from build123d import *

# Parameters (mm, degrees)
SKETCH1_R                = 2.15
BOSS_EXTRUDE1_DEPTH      = 8
BOSS_EXTRUDE2_START      = -4
BOSS_EXTRUDE2_DEPTH      = 4
SKETCH3_W                = 56
SKETCH3_H                = 8
BOSS_EXTRUDE6_DEPTH      = 7
BOSS_EXTRUDE4_START      = -8
BOSS_EXTRUDE4_DEPTH      = 8
CUT_EXTRUDE1_DEPTH       = 67.44206881
FILLET4_R                = 8
FILLET3_R                = 4
M3_CLEARANCE_HOLE1_D     = 3.2
M3_CLEARANCE_HOLE1_DEPTH = 8
M3_CLEARANCE_HOLE1_TIP   = 0.96137699


with BuildPart() as part:
    # Sketch1 → Boss-Extrude1 (new body)
    with BuildSketch(Plane.XY):
        with BuildLine():
            Line((-46, 10), (46, 10))
            ThreePointArc((46, 10), (56, 0), (46, -10))
            Line((46, -10), (-46, -10))
            ThreePointArc((-46, -10), (-56, 0), (-46, 10))
        make_face()
        with Locations((-46, 0)):
            Circle(SKETCH1_R, mode=Mode.SUBTRACT)
        with Locations((46, 0)):
            Circle(SKETCH1_R, mode=Mode.SUBTRACT)
    extrude(amount=BOSS_EXTRUDE1_DEPTH)

    # Sketch2 → Boss-Extrude2 (add)
    with BuildSketch(Plane.XY.offset(8).offset(BOSS_EXTRUDE2_START)):
        with BuildLine():
            Line((-46, -10), (46, -10))
            ThreePointArc((46, -10), (56, 0), (46, 10))
            Line((46, 10), (-46, 10))
            ThreePointArc((-46, 10), (-56, 0), (-46, -10))
        make_face()
    extrude(amount=BOSS_EXTRUDE2_DEPTH)

    # Sketch3 → Boss-Extrude6 (add)
    with BuildSketch(Plane(origin=(0, 10, 0), x_dir=(1, 0, 0), z_dir=(0, 1, 0))):
        with Locations((0, -4)):
            Rectangle(SKETCH3_W, SKETCH3_H)
    extrude(amount=BOSS_EXTRUDE6_DEPTH)

    # Sketch4 → Boss-Extrude4 (add)
    with BuildSketch(Plane.XY.offset(8).offset(BOSS_EXTRUDE4_START)):
        with BuildLine():
            Line((-46, -10), (46, -10))
            ThreePointArc((46, -10), (50.753025174, -8.798224349), (54.363636364, -5.481750339))
            ThreePointArc((54.363636364, -5.481750339), (0, -34.850373137), (-54.363636364, -5.481750339))
            ThreePointArc((-54.363636364, -5.481750339), (-50.753025174, -8.798224349), (-46, -10))
        make_face()
    extrude(amount=BOSS_EXTRUDE4_DEPTH)

    # Sketch5 → Cut-Extrude1 (cut, through all)
    with BuildSketch(Plane(origin=(0, 0, 0), x_dir=(-1, 0, 0), z_dir=(0, 0, -1))):
        with BuildLine():
            Line((-20.322585041, 0), (20.322585041, 0))
            ThreePointArc((20.322585041, 0), (30.049388036, -7.678512657), (24.83871505, -18.922139303))
            ThreePointArc((24.83871505, -18.922139303), (0, -24.850373137), (-24.83871505, -18.922139303))
            ThreePointArc((-24.83871505, -18.922139303), (-30.049388036, -7.678512657), (-20.322585041, 0))
        make_face()
    extrude(amount=-CUT_EXTRUDE1_DEPTH, mode=Mode.SUBTRACT)

    # Fillet4
    # the kernel refuses this fillet: 8 mm, written as the material it adds along each edge
    with BuildSketch(Plane(origin=(28, 10, 8), x_dir=(0, 1, 0), z_dir=(0, 0, -1))) as fillet4_piece_1:
        with BuildLine():
            CenterArc((8, 7.937253933), FILLET4_R, 180, 82.819244219)
            Line((0, 7.937253933), (-0.16, 7.937253933))
            Line((-0.16, 7.937253933), (-0.16, 0))
            Line((-0.16, 0), (0, -0.16))
            ThreePointArc((0, -0.16), (3.5, -0.16), (6.98, -0.158745079))
            Line((6.98, -0.158745079), (7, 0))
        make_face()
    extrude(amount=8)
    with BuildSketch(Plane(origin=(-28, 10, 0), x_dir=(-1, 0, 0), z_dir=(0, 0, 1))) as fillet4_piece_2:
        with BuildLine():
            CenterArc((7.937253933, -8), FILLET4_R, 90, 82.819244219)
            Line((0, -7), (-0.158745079, -6.98))
            ThreePointArc((-0.158745079, -6.98), (-0.16, -3.5), (-0.16, 0))
            Line((-0.16, 0), (0, 0.16))
            Line((0, 0.16), (7.937253933, 0.16))
            Line((7.937253933, 0.16), (7.937253933, 0))
        make_face()
    extrude(amount=8)

    # Fillet3
    fillet3_edges = [part.edges().sort_by_distance(p)[0] for p in [
        (40.968626967, 10, 8),
        (-54.798224349, 4.753025174, 8),
        (54.798224349, 4.753025174, 8),
        (0, -34.850373137, 8),
        (-30.049388036, -7.678512657, 8),
        (0, -24.850373137, 8),
        (30.049388036, -7.678512657, 8),
        (0, 0, 8),
        (-40.968626967, 10, 8),
        (30.645751311, 12, 8),
        (-30.645751311, 12, 8),
    ]]
    fillet(fillet3_edges, radius=FILLET3_R)

    # M3 Clearance Hole1
    with Locations(Plane(origin=(0, 17, 0), x_dir=(1, 0, 0), z_dir=(0, 1, 0))):
        with Locations((-22, -4), (22, -4)):
            Hole(M3_CLEARANCE_HOLE1_D / 2, depth=M3_CLEARANCE_HOLE1_DEPTH)
            with Locations((0, 0, -(M3_CLEARANCE_HOLE1_DEPTH + M3_CLEARANCE_HOLE1_TIP / 2))):  # 118° drill point
                Cone(0, M3_CLEARANCE_HOLE1_D / 2, M3_CLEARANCE_HOLE1_TIP, mode=Mode.SUBTRACT)


solid = part.part
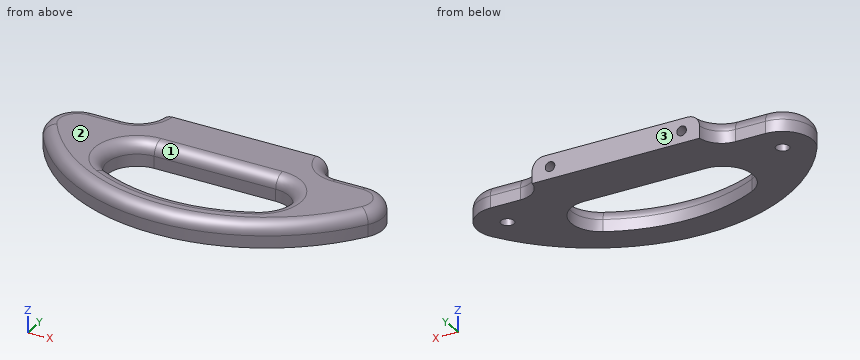
Read the model definition and answer for the solid it produces. Units are mm, in the model's axes. Face numbers are marked on the shaded views. Round coordinates to 2 decimals unless told otherwise and drop trailing zeros.
1) Flat-ended cylindrical pins translate along their axes: pin 1 (4 mm diameter, centred on x = 22, z = 4, fed in from -Y); pin 2 (1.5 mm diameter, centred on y = 8.5, z = 5.5, fed in from -X); pin 3 (4 mm diameter, centred on x = -1, y = -0.5, fed in from +Z). Find the tip coordinate at first contact, or state that the pin passes through.
2) The mould has two halves that part along Y. Classify the marked faces 1, 2 and 3: released by +Y, released by -Y, zero draft, split by the parting line, or undercut.
3) Straight lines are drawn through the part: L1, parallel to Z at x = 22, y = 15; L2, parallel to X at y = 12, z = 4; L3, parallel to X at y = 14.5, z = 4. For each, find the intervals that lie inside material, in ascending order.
Resolved:
1. pin 1: stops at y = -31.7
1. pin 2: stops at x = -51.94
1. pin 3: stops at z = 7.12
2. face 1: undercut
2. face 2: zero draft
2. face 3: released by +Y
3. L1: z = 0 to 2.4, 5.6 to 8
3. L2: x = -30.65 to -23.6, -20.4 to 20.4, 23.6 to 30.65
3. L3: x = -28.74 to -23.6, -20.4 to 20.4, 23.6 to 28.74
